Here's the drawing with two shaded views (mm, measured from the low corner). I have some questions. A direction names the side the tool comes from. Round coordinates to 2 decimals unless told otherwise and drop trailing zeros. Write each loop counter-clockwise with the first axis right and the second up, starting at its lowest first coordinate (ties: lowest second). Pieces come first, ordered by that corner, then holes. Notation, with made-up numbers: M 6,-39 L 63,-39 A25 cw 63,-1 Z; hole C 3,56.5 d7. An arc over 180 degrees is marked long. Write item = value, one per line. Start each with the question number.
(1) If we mould it in two halves opening along Z, with no side actions, what happens to the marked faces 1, 2 and 3? For each: released by +Z, released by -Z, zero draft, split by the parting line, or undercut.
(2) I want a section at B-B (y = 6). List the corners of the cut face in (x, z) for me.
(3) On a 3-axis mill with a long thin cutter (end or side, diameter ignored), from which of +Z, -Z, +X, -X, +Y, -Y can I reach the whole of each face in a straight line? I mean the marked faces 4 and 5. Say none if no direction works.
(4) Will these pins go through, and if not, where does the flat tip stop? pin 1 Ø4 at (x, y) = (3, 1.5) entering from +Z; pin 2 Ø1 at (x, z) = (5.5, 9) entering from +Y; pin 3 Ø2.5 at (y, z) = (6, 6) entering from +X.
(5) I need wall thicknesses on line 1 along Y through (x, z) = (4.4, 6); line 2 along X through (y, z) = (2.75, 7.25); line 3 along Z through (x, y) = (7.25, 6.5). Which ranges of each line are inside material? Lowest first, please.
(6) I want a section at C-C (x = 1.25). List the corners of the cut face in (y, z) for me, and give its area (3 significant figures).
(7) I want a section at D-D (y = 4.5). List the corners of the cut face in (x, z) for me.
(8) I want a section at A-A (z = 6). List the corners of the cut face in (x, y) for me.
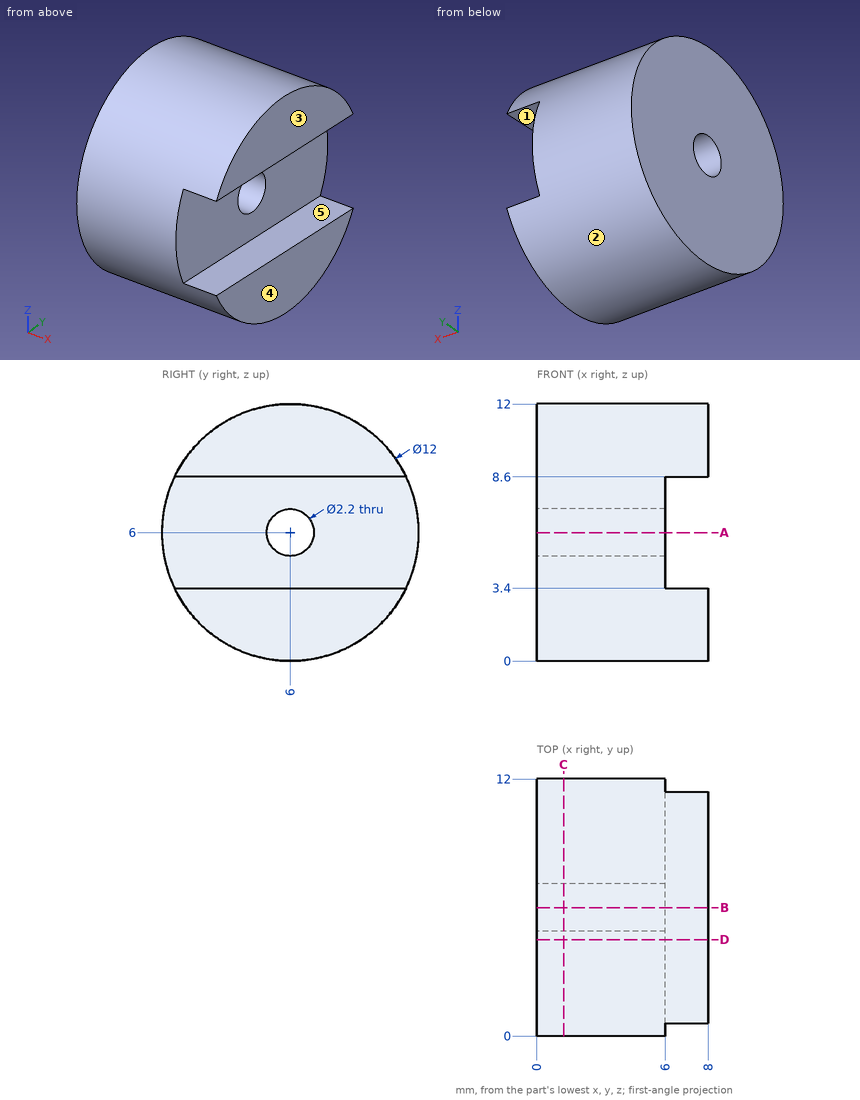
Returned:
q1.face_1 = undercut
q1.face_2 = split by the parting line
q1.face_3 = zero draft
q2.outline = M 0,0 L 8,0 L 8,3.4 L 6,3.4 L 6,4.9 L 0,4.9 Z; M 0,7.1 L 6,7.1 L 6,8.6 L 8,8.6 L 8,12 L 0,12 Z
q3.face_4 = +Z, -Z, +X, +Y, -Y
q3.face_5 = +X, +Y, -Y
q4.pin_1 = 11.45
q4.pin_2 = 11.45
q4.pin_3 = 6
q5.line_1 = 0 to 4.9, 7.1 to 12
q5.line_2 = 0 to 6
q5.line_3 = 0.02 to 3.4, 8.6 to 11.98
q6.outline = C 6,6 d12; hole C 6,6 d2.2
q6.area = 109 mm²
q7.outline = M 0,0.19 L 8,0.19 L 8,3.4 L 6,3.4 L 6,8.6 L 8,8.6 L 8,11.81 L 0,11.81 Z
q8.outline = M 0,0 L 6,0 L 6,4.9 L 0,4.9 Z; M 0,7.1 L 6,7.1 L 6,12 L 0,12 Z
